from build123d import *

# Parameters (mm, degrees)
BOSS_EXTRUDE1_DEPTH = 5
CUT_EXTRUDE1_REACH  = 47.346
SKETCH2_R           = 1.75
SKETCH4_W           = 40
SKETCH4_H           = 35
BOSS_EXTRUDE2_DEPTH = 5
CUT_EXTRUDE2_REACH  = 69.454
SKETCH3_R           = 1.5
SKETCH3_W           = 23.5
SKETCH3_H           = 13.2
FILLET1_R           = 10
FILLET2_R           = 5
FILLET4_R           = 15
BOSS_EXTRUDE3_DEPTH = 6


with BuildPart() as part:
    # Sketch1 → Boss-Extrude1 (new body)
    with BuildSketch(Plane(origin=(0, 0, 0), x_dir=(0, 0, -1), z_dir=(1, 0, 0))):
        with BuildLine():
            ThreePointArc((-25, -12.5), (0, -37.5), (25, -12.5))
            Line((25, -12.5), (25, 12.5))
            Line((25, 12.5), (-25, 12.5))
            Line((-25, 12.5), (-25, -12.5))
        make_face()
    extrude(amount=BOSS_EXTRUDE1_DEPTH)

    # Sketch2 → Cut-Extrude1 (cut, up to next)
    with BuildSketch(Plane(origin=(5, 0, 0), x_dir=(0, 0, -1), z_dir=(1, 0, 0)), mode=Mode.PRIVATE) as cut_extrude1_sk1:
        with Locations((-15, -25.5)):
            Circle(SKETCH2_R)
    cut_extrude1_tool1 = extrude(cut_extrude1_sk1.sketch, amount=-CUT_EXTRUDE1_REACH, mode=Mode.PRIVATE) & part.part
    # Sketch2 → Cut-Extrude1 (cut, up to next)
    with BuildSketch(Plane(origin=(5, 0, 0), x_dir=(0, 0, -1), z_dir=(1, 0, 0)), mode=Mode.PRIVATE) as cut_extrude1_sk2:
        with Locations((15, -25.5)):
            Circle(SKETCH2_R)
    cut_extrude1_tool2 = extrude(cut_extrude1_sk2.sketch, amount=-CUT_EXTRUDE1_REACH, mode=Mode.PRIVATE) & part.part
    # Sketch2 → Cut-Extrude1 (cut, up to next)
    with BuildSketch(Plane(origin=(5, 0, 0), x_dir=(0, 0, -1), z_dir=(1, 0, 0)), mode=Mode.PRIVATE) as cut_extrude1_sk3:
        with Locations((-15, 4.5)):
            Circle(SKETCH2_R)
    cut_extrude1_tool3 = extrude(cut_extrude1_sk3.sketch, amount=-CUT_EXTRUDE1_REACH, mode=Mode.PRIVATE) & part.part
    # Sketch2 → Cut-Extrude1 (cut, up to next)
    with BuildSketch(Plane(origin=(5, 0, 0), x_dir=(0, 0, -1), z_dir=(1, 0, 0)), mode=Mode.PRIVATE) as cut_extrude1_sk4:
        with Locations((0, 4.5)):
            Circle(SKETCH2_R)
    cut_extrude1_tool4 = extrude(cut_extrude1_sk4.sketch, amount=-CUT_EXTRUDE1_REACH, mode=Mode.PRIVATE) & part.part
    # Sketch2 → Cut-Extrude1 (cut, up to next)
    with BuildSketch(Plane(origin=(5, 0, 0), x_dir=(0, 0, -1), z_dir=(1, 0, 0)), mode=Mode.PRIVATE) as cut_extrude1_sk5:
        with Locations((15, 4.5)):
            Circle(SKETCH2_R)
    cut_extrude1_tool5 = extrude(cut_extrude1_sk5.sketch, amount=-CUT_EXTRUDE1_REACH, mode=Mode.PRIVATE) & part.part
    # Sketch2 → Cut-Extrude1 (cut, up to next)
    with BuildSketch(Plane(origin=(5, 0, 0), x_dir=(0, 0, -1), z_dir=(1, 0, 0)), mode=Mode.PRIVATE) as cut_extrude1_sk6:
        with Locations((0, -25.5)):
            Circle(SKETCH2_R)
    cut_extrude1_tool6 = extrude(cut_extrude1_sk6.sketch, amount=-CUT_EXTRUDE1_REACH, mode=Mode.PRIVATE) & part.part
    # Sketch2 → Cut-Extrude1 (cut, up to next)
    with BuildSketch(Plane(origin=(5, 0, 0), x_dir=(0, 0, -1), z_dir=(1, 0, 0)), mode=Mode.PRIVATE) as cut_extrude1_sk7:
        with Locations((-15, -10.5)):
            Circle(SKETCH2_R)
    cut_extrude1_tool7 = extrude(cut_extrude1_sk7.sketch, amount=-CUT_EXTRUDE1_REACH, mode=Mode.PRIVATE) & part.part
    # Sketch2 → Cut-Extrude1 (cut, up to next)
    with BuildSketch(Plane(origin=(5, 0, 0), x_dir=(0, 0, -1), z_dir=(1, 0, 0)), mode=Mode.PRIVATE) as cut_extrude1_sk8:
        with Locations((15, -10.5)):
            Circle(SKETCH2_R)
    cut_extrude1_tool8 = extrude(cut_extrude1_sk8.sketch, amount=-CUT_EXTRUDE1_REACH, mode=Mode.PRIVATE) & part.part
    add(cut_extrude1_tool1.solids().sort_by_distance((5, -25.5, 15))[0], mode=Mode.SUBTRACT)
    add(cut_extrude1_tool2.solids().sort_by_distance((5, -25.5, -15))[0], mode=Mode.SUBTRACT)
    add(cut_extrude1_tool3.solids().sort_by_distance((5, 4.5, 15))[0], mode=Mode.SUBTRACT)
    add(cut_extrude1_tool4.solids().sort_by_distance((5, 4.5, 0))[0], mode=Mode.SUBTRACT)
    add(cut_extrude1_tool5.solids().sort_by_distance((5, 4.5, -15))[0], mode=Mode.SUBTRACT)
    add(cut_extrude1_tool6.solids().sort_by_distance((5, -25.5, 0))[0], mode=Mode.SUBTRACT)
    add(cut_extrude1_tool7.solids().sort_by_distance((5, -10.5, 15))[0], mode=Mode.SUBTRACT)
    add(cut_extrude1_tool8.solids().sort_by_distance((5, -10.5, -15))[0], mode=Mode.SUBTRACT)

    # Sketch4 → Boss-Extrude2 (add)
    with BuildSketch(Plane(origin=(0, 12.5, 0), x_dir=(1, 0, 0), z_dir=(0, 1, 0))):
        with Locations((20, 0)):
            Rectangle(SKETCH4_W, SKETCH4_H)
    extrude(amount=BOSS_EXTRUDE2_DEPTH)

    # Sketch3 → Cut-Extrude2 (cut, up to next)
    with BuildSketch(Plane(origin=(30, 17.5, 0), x_dir=(0, 0, -1), z_dir=(0, 1, 0)), mode=Mode.PRIVATE) as cut_extrude2_sk1:
        with Locations(Location((13.9, 10, 0), (0, 0, 180))):
            Circle(SKETCH3_R)
    cut_extrude2_tool1 = extrude(cut_extrude2_sk1.sketch, amount=-CUT_EXTRUDE2_REACH, mode=Mode.PRIVATE) & part.part
    # Sketch3 → Cut-Extrude2 (cut, up to next)
    with BuildSketch(Plane(origin=(30, 17.5, 0), x_dir=(0, 0, -1), z_dir=(0, 1, 0)), mode=Mode.PRIVATE) as cut_extrude2_sk2:
        with Locations(Location((-13.9, 10, 0), (0, 0, 180))):
            Circle(SKETCH3_R)
    cut_extrude2_tool2 = extrude(cut_extrude2_sk2.sketch, amount=-CUT_EXTRUDE2_REACH, mode=Mode.PRIVATE) & part.part
    # Sketch3 → Cut-Extrude2 (cut, up to next)
    with BuildSketch(Plane(origin=(30, 17.5, 0), x_dir=(0, 0, -1), z_dir=(0, 1, 0)), mode=Mode.PRIVATE) as cut_extrude2_sk3:
        with Locations((0, 10)):
            Rectangle(SKETCH3_W, SKETCH3_H)
    cut_extrude2_tool3 = extrude(cut_extrude2_sk3.sketch, amount=-CUT_EXTRUDE2_REACH, mode=Mode.PRIVATE) & part.part
    add(cut_extrude2_tool1.solids().sort_by_distance((20, 17.5, -13.9))[0], mode=Mode.SUBTRACT)
    add(cut_extrude2_tool2.solids().sort_by_distance((20, 17.5, 13.9))[0], mode=Mode.SUBTRACT)
    add(cut_extrude2_tool3.solids().sort_by_distance((20, 17.5, 0))[0], mode=Mode.SUBTRACT)

    # Fillet1
    fillet1_edges = [part.edges().sort_by_distance(p)[0] for p in [
        (40, 15, 17.5),
        (40, 15, -17.5),
    ]]
    fillet(fillet1_edges, radius=FILLET1_R)

    # Fillet2
    fillet2_edges = [part.edges().sort_by_distance(p)[0] for p in [
        (0, 17.5, 0),
    ]]
    fillet(fillet2_edges, radius=FILLET2_R)

    # Fillet4
    # the kernel refuses this fillet: 15 mm, written as the material it takes off along each edge
    with BuildSketch(Plane(origin=(-32.475952642, 12.5, 25), x_dir=(0, 0, -1), z_dir=(1, 0, 0))) as fillet4_piece_1:
        with BuildLine():
            CenterArc((15, -12.990381057), FILLET4_R, 120, 60)
            Line((0, -12.990381057), (-0.3, -12.990381057))
            Line((-0.3, -12.990381057), (-0.3, 0))
            Line((-0.3, 0), (0, 0.3))
            ThreePointArc((0, 0.3), (3.75, 0.3), (7.35, 0.259807621))
            Line((7.35, 0.259807621), (7.5, 0))
        make_face()
    extrude(amount=69.951905284, mode=Mode.SUBTRACT)
    with BuildSketch(Plane(origin=(-32.475952642, 12.5, -25), x_dir=(0, 0, 1), z_dir=(1, 0, 0))) as fillet4_piece_2:
        with BuildLine():
            CenterArc((15, 12.990381057), FILLET4_R, 180, 60)
            Line((0, 12.990381057), (-0.3, 12.990381057))
            Line((-0.3, 12.990381057), (-0.3, 0))
            Line((-0.3, 0), (0, -0.3))
            ThreePointArc((0, -0.3), (3.75, -0.3), (7.35, -0.259807621))
            Line((7.35, -0.259807621), (7.5, 0))
        make_face()
    extrude(amount=69.951905284, mode=Mode.SUBTRACT)

    # Sketch5 → Boss-Extrude3 (add)
    with BuildSketch(Plane(origin=(0, 0, -17.5), x_dir=(-1, 0, 0), z_dir=(0, 0, -1))):
        Polygon((-5, 6.5), (-5, 12.5), (-12, 12.5), align=None)
    boss_extrude3 = extrude(amount=-BOSS_EXTRUDE3_DEPTH)

    # Mirror1: Boss-Extrude3 across plane
    add(boss_extrude3.mirror(Plane.XY))


solid = part.part
Input: part model. Units: mm. Frame: model coordinates. A direction names the side the tool comes from. Coordinates: 2 decimals unless noted, no trailing zeros. Order: outer loops, then holes, each group sorted by start corner. A loop starts at its lowest first (then second) coordinate and runs counter-clockwise, first axis right, second up. Notation, with made-up numbers: M 46.25,-17.75 L 78.25,-17.75 A14 ccw 78.25,-10.75 Z; hole C 65,29 d10. An arc over 180 degrees is marked long. Answer as CSV lines item,"result".
1. First-contact query: P1, Ø4.5, axis at y = -10.5, z = 15, coming from the +X side; P2, Ø6.5, axis at x = 8.5, y = 8, coming from the +Z side; P3, Ø2, axis at x = 25, z = -16.5, coming from the -Y side. Flat tips, straight axial feed; report the tip coordinate or a pass-through.
Reported:
P1,"x = 5"
P2,"z = 17.5"
P3,"y = 12.5"
2. Pull-direction query (Z, two-part tool) for faces 3 (the cylindrical face through (36.99, 15.04, 14.65)), 4 (the cylindrical face through (2.465, 6.914, -23.045)), 5 (the cylindrical face through (21.01, 15.04, 12.79)), 6 (the flat face through (8.5, 9.5, 14.5)); classes: released by +Z, released by -Z, zero draft, split by the parting line, or undercut.
Reported:
face 3,"released by +Z"
face 4,"released by -Z"
face 5,"undercut"
face 6,"zero draft"
3. Section D-D (x = 4). State how many separate pieces and enclosed holes the cut face has, then the cut area to 3 significant figures.
Reported:
separate pieces,"1"
enclosed holes,"8"
area,"2,270 mm2"
4. Section C-C (z = 5). Return the cut outline in (x, y), then the cut area to 3 significant figures.
Reported:
outline,"M 0,-36.99 L 5,-36.99 L 5,12.5 L 13.4,12.5 L 13.4,17.5 L 5,17.5 A5 ccw 0,12.5 Z; M 26.6,12.5 L 40,12.5 L 40,17.5 L 26.6,17.5 Z"
area,"376 mm2"
5. Section B-B (y = -25.5). Return the cut outline in (x, z).
Reported:
outline,"M 0,-21.35 L 5,-21.35 L 5,-16.75 L 0,-16.75 Z; M 0,-13.25 L 5,-13.25 L 5,-1.75 L 0,-1.75 Z; M 0,1.75 L 5,1.75 L 5,13.25 L 0,13.25 Z; M 0,16.75 L 5,16.75 L 5,21.35 L 0,21.35 Z"
6. Access query for faces 1 (the flat face through (30, 12.5, 0)), 2 (the cylindrical face through (2.54, 2.95, -15.81)). Directions: +Z, -Z, +X, -X, +Y, -Y. A direction counts if a zero-diameter tool reaches every point of the face in a straight line with its end or side. Return the directions, or none.
Reported:
face 1,"+X, -Y"
face 2,"+X, -X"
7. Section A-A (x = 16). Return the cut outline in (y, z).
Reported:
outline,"M 12.5,-17.5 L 17.5,-17.5 L 17.5,-11.75 L 12.5,-11.75 Z; M 12.5,11.75 L 17.5,11.75 L 17.5,17.5 L 12.5,17.5 Z"
8. Material intervals for line 1 (Y direction, x = 2, z = 15); line 2 (Y direction, x = 1.6, z = 0); line 3 (Y direction, x = 1, z = -15), sorted ascending. Write a range as from..to.
Reported:
line 1,"-32.5..-27.25, -23.75..-12.25, -8.75..2.75, 6.25..16.5"
line 2,"-37.5..-27.25, -23.75..2.75, 6.25..16.17"
line 3,"-32.5..-27.25, -23.75..-12.25, -8.75..2.75, 6.25..15.5"
